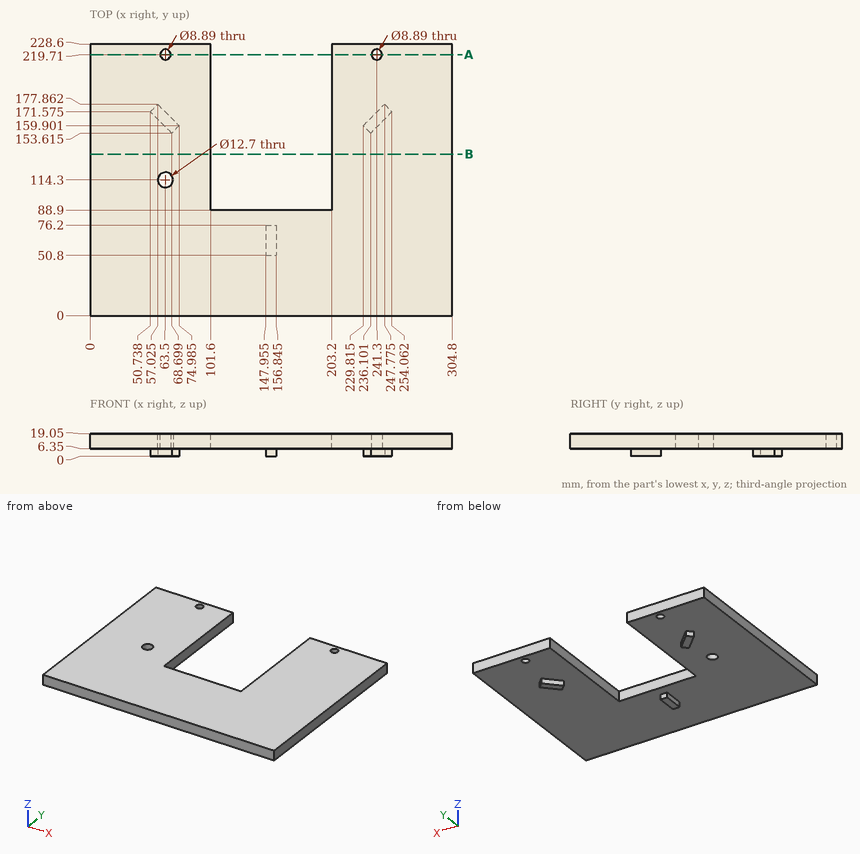
Verification items for this drawing (mm, ordinates from the low corner). Round coordinates to 2 decimals unless told otherwise and drop trailing zeros. Loops run counter-clockwise (first coordinate to the right, second up) from the corner with the lowest first, then second, coordinate; pieces in that order, holes last. Notation, with made-up numbers: (44.25, 70.25) - (72.25, 70.25) arc R25 cw to (72.25, 93.25) - close; hole circle Ø9 at (34.25, 49.25). An arc over 180 degrees is marked (long way). Write item = value, one per line.
Q1. Depth check by flat-ended pin: pin 1 (6 mm diameter, centred on x = 167.5, z = 12.5, fed in from +Y); pin 2 (7 mm diameter, centred on x = 63.5, y = 219.71, fed in from -Z); pin 3 (5 mm diameter, centred on y = 68, z = 1.5, fed in from -X) (3 decimals); pin 4 (1.9 mm diameter, centred on y = 66.5, z = 1.5, fed in from +X) (3 decimals). Enter the tip coordinate at first touch or a pass-through.
Here are the results:
pin_1 = 88.9
pin_2 = through
pin_3 = 147.955
pin_4 = 156.845
Q2. Sectioned sample at A-A on y = 219.71. State how many separate pieces and enclosed holes the cut face has.
Here are the results:
separate_pieces = 4
enclosed_holes = 0
Q3. Material ranges on L1, parallel to X at y = 219.71, z = 15.25 (1 decimal); L2, parallel to Y at x = 241.3, z = 10 (1 decimal); L3, parallel to Y at x = 171, z = 8.5, recorded low to high.
Here are the results:
L1 = 0 to 59.1, 67.9 to 101.6, 203.2 to 236.9, 245.7 to 304.8
L2 = 0 to 215.3, 224.2 to 228.6
L3 = 0 to 88.9
Q4. Sectioned sample at B-B on y = 136. Record the boundary of the cut face in (x, z), plus the area to 3 significant figures.
Here are the results:
outline = (0, 6.35) - (101.6, 6.35) - (101.6, 19.05) - (0, 19.05) - close; (203.2, 6.35) - (304.8, 6.35) - (304.8, 19.05) - (203.2, 19.05) - close
area = 2,580 mm^2
